```python
from build123d import *

# Parameters (mm, degrees)
SKETCH_LID_W                 = 80
SKETCH_LID_H                 = 50
BOSS_EXTRUDE_LID_DEPTH       = 2
FILLET_CORNERS_R             = 7
SKETCH_SCREW_HOLE_R          = 2
CUT_EXTRUDE_SCREW_HOLE_DEPTH = 2


with BuildPart() as part:
    # Sketch_lid → Boss-Extrude_lid (new body)
    with BuildSketch(Plane(origin=(0, 0, 0), x_dir=(1, 0, 0), z_dir=(0, 1, 0))):
        Rectangle(SKETCH_LID_W, SKETCH_LID_H)
    extrude(amount=BOSS_EXTRUDE_LID_DEPTH)

    # Fillet_corners
    fillet_corners_edges = [part.edges().sort_by_distance(p)[0] for p in [
        (40, 1, 25),
        (-40, 1, 25),
        (-40, 1, -25),
        (40, 1, -25),
    ]]
    fillet(fillet_corners_edges, radius=FILLET_CORNERS_R)

    # Sketch_screw_hole → Cut-Extrude_screw_hole (cut)
    with BuildSketch(Plane.XZ):
        with Locations(Location((-35, -20, 0), (0, 0, 270))):
            Circle(SKETCH_SCREW_HOLE_R)
        with Locations(Location((35, -20, 0), (0, 0, 270))):
            Circle(SKETCH_SCREW_HOLE_R)
        with Locations(Location((35, 20, 0), (0, 0, 270))):
            Circle(SKETCH_SCREW_HOLE_R)
        with Locations(Location((-35, 20, 0), (0, 0, 270))):
            Circle(SKETCH_SCREW_HOLE_R)
    extrude(amount=-CUT_EXTRUDE_SCREW_HOLE_DEPTH, mode=Mode.SUBTRACT)


solid = part.part
```
Geometry: final body of the model. Coordinates: model frame, mm. Give positions to 0.01 mm unless a question says otherwise; leave off trailing zeros. Loops run counter-clockwise (first coordinate to the right, second up) from the corner with the lowest first, then second, coordinate; pieces in that order, holes last. Notation, with made-up numbers: (70.25, -27.5) -> (118.25, -27.5) arc R28 ccw to (118.25, 8.5) -> close; hole circle Ø4 at (0.25, 76.25). An arc over 180 degrees is marked (long way). Return JSON: item names as keys, results as strings.
Item 1: Section C-C, the plane x = -35. Output: boundary loops of the cut face in (y, z), plus the area to 3 significant figures.
Filled in:
{"outline": "(0, -24.71) -> (2, -24.71) -> (2, -22) -> (0, -22) -> close; (0, -18) -> (2, -18) -> (2, 18) -> (0, 18) -> close; (0, 22) -> (2, 22) -> (2, 24.71) -> (0, 24.71) -> close", "area": "82.8 mm^2"}
Item 2: Mould query, pull axis Z, two halves, no side actions, for faces 1 (the flat face through (0, 1, 25)), 2 (the flat face through (-1, 2, 0)), 3 (the cylindrical face through (-37, 1, -20)). Classes: released by +Z, released by -Z, zero draft, split by the parting line, or undercut.
Filled in:
{"face 1": "released by +Z", "face 2": "zero draft", "face 3": "undercut"}
Item 3: Section B-B, the plane z = 20. Output: boundary loops of the cut face in (x, y).
Filled in:
{"outline": "(-39.71, 0) -> (-37, 0) -> (-37, 2) -> (-39.71, 2) -> close; (-33, 0) -> (33, 0) -> (33, 2) -> (-33, 2) -> close; (37, 0) -> (39.71, 0) -> (39.71, 2) -> (37, 2) -> close"}
Item 4: Section A-A, the plane y = 0.45. Output: boundary loops of the cut face in (x, z).
Filled in:
{"outline": "(-40, -18) arc R7 ccw to (-33, -25) -> (33, -25) arc R7 ccw to (40, -18) -> (40, 18) arc R7 ccw to (33, 25) -> (-33, 25) arc R7 ccw to (-40, 18) -> close; hole circle Ø4 at (-35, -20); hole circle Ø4 at (-35, 20); hole circle Ø4 at (35, -20); hole circle Ø4 at (35, 20)"}
Item 5: Line query: line 1 (Z direction, x = -34, y = 0.4); line 2 (X direction, y = 1.4, z = 20); line 3 (Z direction, x = -36, y = 1.4). Output: solid intervals per line, ascending.
Filled in:
{"line 1": "-24.93 to -21.73, -18.27 to 18.27, 21.73 to 24.93", "line 2": "-39.71 to -37, -33 to 33, 37 to 39.71", "line 3": "-24.32 to -21.73, -18.27 to 18.27, 21.73 to 24.32"}
